Check sheet for the modelled part. Datum: model origin and axes. Units: mm. Face numbers are marked on the shaded views. A direction names the side the tool comes from. Coordinates: 2 decimals unless noted, no trailing zeros. Order: outer loops, then holes, each group sorted by start corner. A loop starts at its lowest first (then second) coordinate and runs counter-clockwise, first axis right, second up.
from build123d import *

# Parameters (mm, degrees)
SKETCH1_W            = 50.8
SKETCH1_H            = 50.8
SKETCH1_W_2          = 44.45
SKETCH1_H_2          = 44.45
BOSS_EXTRUDE1_DEPTH  = 101.6
SKETCH2_R            = 3.429
CUT_EXTRUDE1_DEPTH   = 101.6
LPATTERN1_COUNT      = 3
LPATTERN1_PITCH      = 12.7
LPATTERN1_COUNT_DIR2 = 2
LPATTERN1_PITCH_DIR2 = 19.05


with BuildPart() as part:
    # Sketch1 → Boss-Extrude1 (new body)
    with BuildSketch(Plane(origin=(0, 0, 0), x_dir=(1, 0, 0), z_dir=(0, 1, 0))):
        Rectangle(SKETCH1_W, SKETCH1_H)
        Rectangle(SKETCH1_W_2, SKETCH1_H_2, mode=Mode.SUBTRACT)
    extrude(amount=BOSS_EXTRUDE1_DEPTH)

    # Sketch2 → Cut-Extrude1 (cut)
    with BuildSketch(Plane.XY.offset(25.4)):
        with Locations((-12.7, 69.85)):
            Circle(SKETCH2_R)
    cut_extrude1 = extrude(amount=-CUT_EXTRUDE1_DEPTH, mode=Mode.SUBTRACT)

    # LPattern1: Cut-Extrude1 3 × 2
    with Locations(*[(i * LPATTERN1_PITCH, j * LPATTERN1_PITCH_DIR2, 0) for i in range(LPATTERN1_COUNT) for j in range(LPATTERN1_COUNT_DIR2) if (i, j) != (0, 0)]):
        add(cut_extrude1, mode=Mode.SUBTRACT)


solid = part.part
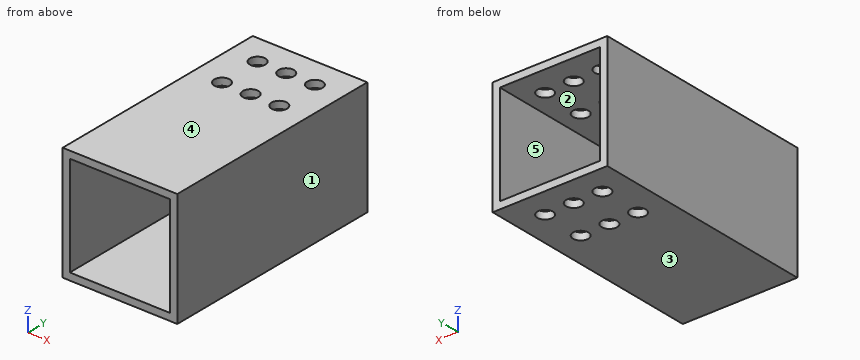
(1) Thickness scan on probe 1 along X at (y, z) = (88.9, -24.2); probe 2 along Y at (x, z) = (0, 23.3); probe 3 along Z at (x, y) = (7, 24) (3 decimals). Record the ranges inside material, lowest first.
Filled in:
probe 1: x = -25.4 to -16.13, -9.27 to -3.43, 3.43 to 9.27, 16.13 to 25.4
probe 2: y = 0 to 66.42, 73.28 to 85.47, 92.33 to 101.6
probe 3: z = -25.4 to -22.225, 22.225 to 25.4
(2) Go/stop test with a flat-tipped pin: P1, Ø9, axis at x = -12.7, y = 88.9, coming from the -Z side. Record where the tip stops, or that it passes through.
Filled in:
P1: stops at z = -25.4
(3) Release check for a two-part mould opening along Z. For the marked faces 3, 4 and 5 record: +Z half, -Z half, draft (parallel to the pull), parting line (faces both ways), or undercut.
Filled in:
face 3: -Z half
face 4: +Z half
face 5: undercut
(4) Cross-section at D-D (y = 46.5). Enter the section's corners in (x, z) (3 decimals).
Filled in:
outline: (-25.4, -25.4) - (25.4, -25.4) - (25.4, 25.4) - (-25.4, 25.4) - close; hole (-22.225, -22.225) - (22.225, -22.225) - (22.225, 22.225) - (-22.225, 22.225) - close
(5) Cross-section at A-A (z = 12). Enter the section's corners in (x, y) (3 decimals).
Filled in:
outline: (-25.4, 0) - (-22.225, 0) - (-22.225, 101.6) - (-25.4, 101.6) - close; (22.225, 0) - (25.4, 0) - (25.4, 101.6) - (22.225, 101.6) - close
(6) Tool access check on the marked faces 1 and 2. Record the directions out of +Z, -Z, +X, -X, +Y, -Y that give a thin tool (end or side, any length) a straight path to the whole face; none if there is none.
Filled in:
face 1: +Z, -Z, +X, +Y, -Y
face 2: +Y, -Y
(7) Cross-section at B-B (x = -5). Enter the section's corners in (y, z) (3 decimals), and give its area (3 significant figures).
Filled in:
outline: (0, -25.4) - (101.6, -25.4) - (101.6, -22.225) - (0, -22.225) - close; (0, 22.225) - (101.6, 22.225) - (101.6, 25.4) - (0, 25.4) - close
area: 645 mm2
(8) Cross-section at C-C (y = 69.85). Count the separate pieces of the cut face and the enclosed holes in it, and give its area (3 significant figures).
Filled in:
separate pieces: 6
enclosed holes: 0
area: 474 mm2
